from build123d import *

# Parameters (mm, degrees)
SKETCH1_R           = 2.325
SKETCH1_W           = 7.749999992
SKETCH1_H           = 9.652
BOSS_EXTRUDE1_DEPTH = 12.7
SKETCH2_R           = 4.826
CUT_EXTRUDE1_DEPTH  = 8


with BuildPart() as part:
    # Sketch1 → Boss-Extrude1 (new body)
    # profile 1 of 2: a face of its own
    with BuildSketch(Plane.XY):
        Polygon((90.626647956, 23.365008212), (81.539999992, 23.365008212), (81.539999992, -23.365008212), (90.626647956, -23.365008212), (94.239999992, -17.607359271), (94.239999992, -4.826), (86.49, -4.826), (86.49, 4.826), (94.239999992, 4.826), (94.239999992, 17.607359271), align=None)
        with Locations((89.96, -15)):
            Circle(SKETCH1_R, mode=Mode.SUBTRACT)
        with Locations((89.96, 15)):
            Circle(SKETCH1_R, mode=Mode.SUBTRACT)
    # profile 2 of 2: a face of its own
    with BuildSketch(Plane.XY):
        with Locations((90.364999996, 0)):
            Rectangle(SKETCH1_W, SKETCH1_H)
    extrude(amount=BOSS_EXTRUDE1_DEPTH)

    # Sketch2 → Cut-Extrude1 (cut)
    with BuildSketch(Plane(origin=(94.239999992, 0, 0), x_dir=(0, 0, -1), z_dir=(1, 0, 0))):
        Circle(SKETCH2_R)
    extrude(amount=-CUT_EXTRUDE1_DEPTH, mode=Mode.SUBTRACT)


solid = part.part
Geometry: final body of the model. Coordinates: model frame, mm. A direction names the side the tool comes from. Give positions to 0.01 mm unless a question says otherwise; leave off trailing zeros. Write each loop counter-clockwise with the first axis right and the second up, starting at its lowest first coordinate (ties: lowest second). Pieces come first, ordered by that corner, then holes.
(1) Mould query, pull axis Y, two halves, no side actions, for faces 1 (the flat face through (86.24, 0, 2)), 2 (the flat face through (92.459, 20.446, 6.261)), 3 (the flat face through (94.24, 0, 6)). Classes: released by +Y, released by -Y, zero draft, split by the parting line, or undercut.
(2) Ray query, line 1 (Y direction, x = 89.96, z = 5.75) (3 decimals); line 2 (Y direction, x = 90, z = 4) (3 decimals); line 3 (Y direction, x = 89.96, z = 3) (3 decimals). Return the intervals inside material, ascending.
(3) Access query for faces 4 (the flat face through (81.54, 0, 6)), 5 (the cylindrical face through (90.296, 0.106, 4.825)). Directions: +Z, -Z, +X, -X, +Y, -Y. A direction counts if a zero-diameter tool reaches every point of the face in a straight line with its end or side. Return the directions, or none.
(4) Cut plane A-A, the plane z = 5.5. Return loops of the section in (x, y) (3 decimals).
(5) Cut plane C-C, the plane x = 86.75. Return loops of the section in (y, z) (3 decimals).
(6) First-contact query: P1, Ø6, axis at x = 92, z = 9.5, coming from the -Y side (3 decimals). Flat tip, straight axial feed; report the tip coordinate or a pass-through.
(7) Cut plane B-B, the plane y = 15. Return loops of the section in (x, z) (3 decimals).
(8) Cut plane D-D, the plane y = 0. Return loops of the section in (x, z).
Values follow:
1. face 1: undercut
1. face 2: released by +Y
1. face 3: zero draft
2. line 1: y = -23.365 to -17.325, -12.675 to 12.675, 17.325 to 23.365
2. line 2: y = -23.365 to -17.325, -12.675 to -2.7, 2.7 to 12.675, 17.325 to 23.365
2. line 3: y = -23.365 to -17.325, -12.675 to -3.78, 3.78 to 12.675, 17.325 to 23.365
3. face 4: +Z, -Z, -X, +Y, -Y
3. face 5: -Z, +X
4. outline: (81.54, -23.365) - (90.627, -23.365) - (94.24, -17.607) - (94.24, 17.607) - (90.627, 23.365) - (81.54, 23.365) - close; hole circle Ø4.65 at (89.96, -15); hole circle Ø4.65 at (89.96, 15)
5. outline: (-23.365, 0) - (-4.826, 0) arc R4.826 cw to (4.826, 0) - (23.365, 0) - (23.365, 12.7) - (-23.365, 12.7) - close
6. P1: stops at y = -23.365
7. outline: (81.54, 0) - (87.635, 0) - (87.635, 12.7) - (81.54, 12.7) - close; (92.285, 0) - (94.24, 0) - (94.24, 12.7) - (92.285, 12.7) - close
8. outline: (81.54, 0) - (86.24, 0) - (86.24, 4.83) - (94.24, 4.83) - (94.24, 12.7) - (81.54, 12.7) - close
